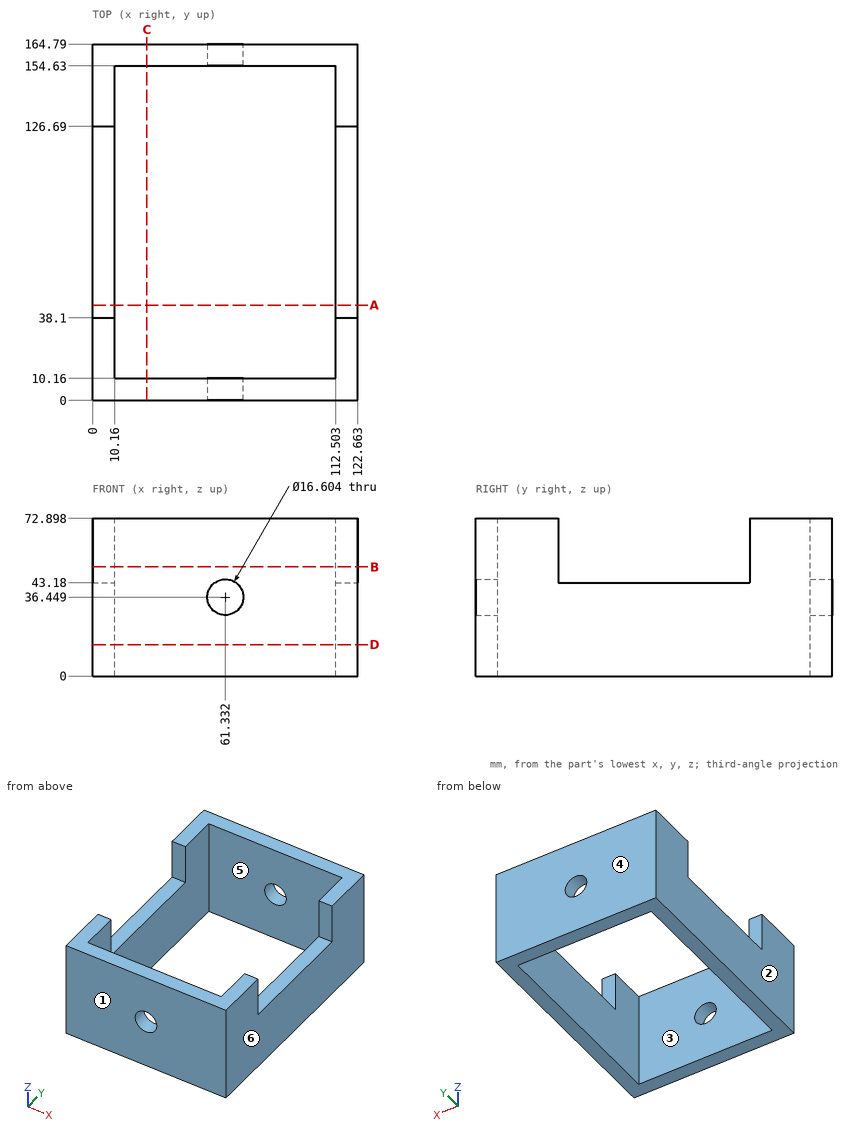
Input: dimensioned drawing with shaded views. Units: mm. Origin: part minimum x, y, z. A direction names the side the tool comes from. Coordinates: 2 decimals unless noted, no trailing zeros. Order: outer loops, then holes, each group sorted by start corner. A loop starts at its lowest first (then second) coordinate and runs counter-clockwise, first axis right, second up.
(1) Section query C-C (x = 25). Return the cut outline in (y, z), plus the area to 3 significant figures.
(2) Section query B-B (z = 50.5). Return the cut outline in (x, y), plus the area to 3 significant figures.
(3) Material intervals for probe 1 along Y at (x, z) = (95.5, 64); probe 2 along X at (y, z) = (125, 11), sorted ascending.
(4) Access query for the marked faces 5 and 6. Directions: +Z, -Z, +X, -X, +Y, -Y. A direction counts if a zero-diameter tool reaches every point of the face in a straight line with its end or side. Return the directions, or none.
(5) Section query A-A (y = 44). Return the cut outline in (x, z).
(6) Draft query along Y for the marked faces 1, 2, 3 and 4. Return one class per face: pulls with the +Y half, pulls with the -Y half, needs draft (parallel to the pull), parting line crosses it, or undercut.
(7) Section query D-D (z = 14.5). Return the cut outline in (x, y).
(8) First-contact query: pin 1 (5 mm diameter, centred on x = 119.5, y = 83.5, fed in from +Z); pin 2 (13.5 mm diameter, centred on x = 61.33, z = 36.45, fed in from -Y). Flat tips, straight axial feed; report the tip coordinate or a pass-through.
Solution:
1. outline: (0, 0) - (10.16, 0) - (10.16, 72.9) - (0, 72.9) - close; (154.63, 0) - (164.79, 0) - (164.79, 72.9) - (154.63, 72.9) - close
1. area: 1,480 mm2
2. outline: (0, 0) - (122.66, 0) - (122.66, 38.1) - (112.5, 38.1) - (112.5, 10.16) - (10.16, 10.16) - (10.16, 38.1) - (0, 38.1) - close; (0, 126.69) - (10.16, 126.69) - (10.16, 154.63) - (112.5, 154.63) - (112.5, 126.69) - (122.66, 126.69) - (122.66, 164.79) - (0, 164.79) - close
2. area: 3,630 mm2
3. probe 1: y = 0 to 10.16, 154.63 to 164.79
3. probe 2: x = 0 to 10.16, 112.5 to 122.66
4. face 5: +Z, -Z
4. face 6: +Z, -Z, +X, +Y, -Y
5. outline: (0, 0) - (10.16, 0) - (10.16, 43.18) - (0, 43.18) - close; (112.5, 0) - (122.66, 0) - (122.66, 43.18) - (112.5, 43.18) - close
6. face 1: pulls with the -Y half
6. face 2: needs draft
6. face 3: undercut
6. face 4: pulls with the +Y half
7. outline: (0, 0) - (122.66, 0) - (122.66, 164.79) - (0, 164.79) - close; hole (10.16, 10.16) - (112.5, 10.16) - (112.5, 154.63) - (10.16, 154.63) - close
8. pin 1: stops at z = 43.18
8. pin 2: passes through
